CAD build for the part. Positions are in the model's coordinates, mm. Face numbers are marked on the shaded views. Give positions to 0.01 mm unless a question says otherwise; leave off trailing zeros. Write each loop counter-clockwise with the first axis right and the second up, starting at its lowest first coordinate (ties: lowest second). Pieces come first, ordered by that corner, then holes. Notation, with made-up numbers: M 80,25 L 84,25 A15 ccw 84,44 Z; hole C 41.5,17 d8. An arc over 180 degrees is marked long. One line per question, with ' | ' between items. Start each with the question number.
1. Cut at A-A, the plane x = 15. Write the cut outline in (y, z).
2. Cut at C-C, the plane z = 58. Write the cut outline in (x, y), then the cut area to 3 significant figures.
3. Cut at B-B, the plane y = -15. Write the cut outline in (x, z).
4. Cut at D-D, the plane y = -31. Write the cut outline in (x, z), then the cut area to 4 significant figures.
5. Flat gauge pin, fed straight in: pin 1 (10 mm diameter, centred on y = -16, z = 98, fed in from +X). Where does the tip first touch, or does it go through?
6. Wall check: L1, parallel to Z at x = 16.75, y = -19; L2, parallel to X at y = -22.5, z = 55; L3, parallel to X at y = -16, z = 75.5. Give the ranges that are in metal, low to high.
7. Pull direction Z, two halves, no side cores. Call the marked faces 1, 2 and 3: released by +Z, released by -Z, zero draft, split by the parting line, or undercut.
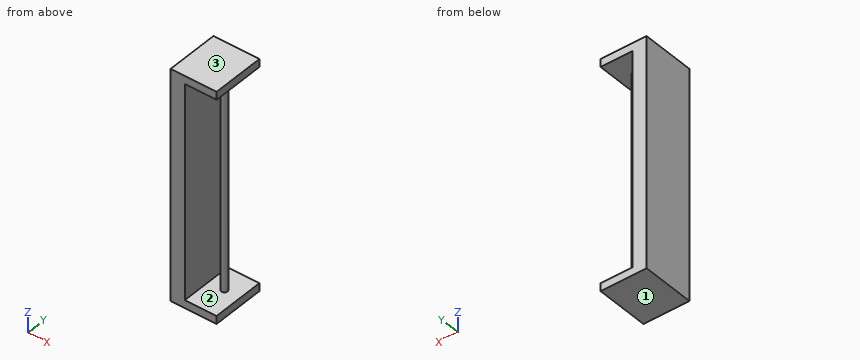
Autodesk Inventor part; units mm, degrees
ref_plane "YZ Plane" through (0, 0, 0) normal (1, 0, 0) x (0, 1, 0)
ref_plane "XZ Plane" through (0, 0, 0) normal (0, 1, 0) x (-1, 0, 0)
ref_plane "XY Plane" through (0, 0, 0) normal (0, 0, 1) x (1, 0, 0)
sketch "스케치1" plane through (0, 0, 0) normal (0, 0, 1) x (1, 0, 0)
  line L0 (0, 0) -> (29, 0)
  line L1 (29, 0) -> (29, -33.5)
  line L2 (29, -33.5) -> (0, -33.5)
  line L3 (0, -33.5) -> (0, 0)
  dimension "d0" = 29
  dimension "d1" = 33.5
extrude "돌출1" add sketch "스케치1" along normal blind 145
sketch "스케치2" plane through (29, -33.5, 0) normal (1, 0, 0) x (0, 0, -1)
  line L0 (0, 0) -> (0, 33.5)
  line L1 (0, 33.5) -> (-145, 33.5)
  line L2 (-145, 0) -> (-145, 33.5)
  line L3 (0, 0) -> (-145, 0)
  line L4 (-140, 33.5) -> (-140, 0)
  line L5 (-5, 33.5) -> (-5, 0)
  dimension "d4" = 5
  dimension "d5" = 5
extrude "돌출2" cut sketch "스케치2" against normal blind 20 contours L3 L4 L1 L5
sketch "스케치3" plane through (29, -33.5, 140) normal (0, 0, -1) x (-1, 0, 0)
  line L0 (0, 0) -> (0, 33.5)
  line L1 (20, 0) -> (0, 0)
  line L2 (20, 0) -> (20, 33.5)
  line L3 (0, 33.5) -> (20, 33.5)
  circle A0 centre (10, 18.5) radius 2
  point P0 (29, 33.5)
  dimension "d8" = 4
  dimension "d9" = 10
  dimension "d10" = 18.5
extrude "돌출3" add sketch "스케치3" along normal up to surface (135 mm away) contours A0
properties part number "linear_motor"
Here are the results:
1) outline: M -33.5,0 L 0,0 L 0,5 L -33.5,5 Z; M -33.5,140 L 0,140 L 0,145 L -33.5,145 Z
2) outline: M 0,-33.5 L 9,-33.5 L 9,0 L 0,0 Z; C 19,-15 d4 | area: 314 mm^2
3) outline: M 0,0 L 29,0 L 29,5 L 21,5 L 21,140 L 29,140 L 29,145 L 0,145 Z; hole M 9,5 L 17,5 L 17,140 L 9,140 Z
4) outline: M 0,0 L 29,0 L 29,5 L 9,5 L 9,140 L 29,140 L 29,145 L 0,145 Z | area: 1,505 mm^2
5) pin 1: x = 21
6) L1: 0 to 5, 140 to 145 | L2: 0 to 9 | L3: 0 to 9, 17.27 to 20.73
7) face 1: released by -Z | face 2: undercut | face 3: released by +Z
